Design review of the part built by this model. Coordinates are the model's own, in mm. A direction names the side the tool comes from. Give positions to 0.01 mm unless a question says otherwise; leave off trailing zeros. Write each loop counter-clockwise with the first axis right and the second up, starting at its lowest first coordinate (ties: lowest second). Pieces come first, ordered by that corner, then holes. Notation, with made-up numbers: (-38, 82.25) -> (16, 82.25) arc R24 cw to (16, 100.25) -> close; hole circle Ø9 at (-22.75, 15). An arc over 180 degrees is marked (long way). Answer as a JSON object with one key per item and string values.
```python
from build123d import *

# Parameters (mm, degrees)
ESQUISSE1_R        = 1.925
BOSS_EXTRU_1_DEPTH = 5


with BuildPart() as part:
    # Esquisse1 → Boss.-Extru.1 (new body)
    with BuildSketch(Plane.XY):
        with BuildLine():
            Line((13.05, 32.5), (-13.05, 32.5))
            ThreePointArc((-13.05, 32.5), (-14.464213562, 31.914213562), (-15.05, 30.5))
            Line((-15.05, 30.5), (-15.05, 25))
            Line((-15.05, 25), (-13.55, 25))
            Line((-13.55, 25), (-13.55, 21))
            Line((-13.55, 21), (-20.45, 21))
            Line((-20.45, 21), (-20.45, 25))
            Line((-20.45, 25), (-18.95, 25))
            Line((-18.95, 25), (-18.95, 30.5))
            ThreePointArc((-18.95, 30.5), (-19.535786438, 31.914213562), (-20.95, 32.5))
            Line((-20.95, 32.5), (-23, 32.5))
            Line((-23, 32.5), (-23, 37.5))
            Line((-23, 37.5), (-25.999999067, 37.497633905))
            ThreePointArc((-25.999999067, 37.497633905), (-26.620839292, 37.398317642), (-27.180168114, 37.111163374))
            ThreePointArc((-27.180168114, 37.111163374), (-45.999999844, 0), (-27.180168114, -37.111163374))
            ThreePointArc((-27.180168114, -37.111163374), (-26.620839292, -37.398317642), (-25.999999067, -37.497633905))
            Line((-25.999999067, -37.497633905), (-23, -37.5))
            Line((-23, -37.5), (-23, -32.5))
            Line((-23, -32.5), (-20.95, -32.5))
            ThreePointArc((-20.95, -32.5), (-19.535786438, -31.914213562), (-18.95, -30.5))
            Line((-18.95, -30.5), (-18.95, -25))
            Line((-18.95, -25), (-20.45, -25))
            Line((-20.45, -25), (-20.45, -21))
            Line((-20.45, -21), (-13.55, -21))
            Line((-13.55, -21), (-13.55, -25))
            Line((-13.55, -25), (-15.05, -25))
            Line((-15.05, -25), (-15.05, -30.5))
            ThreePointArc((-15.05, -30.5), (-14.464213562, -31.914213562), (-13.05, -32.5))
            Line((-13.05, -32.5), (13.05, -32.5))
            ThreePointArc((13.05, -32.5), (14.464213562, -31.914213562), (15.05, -30.5))
            Line((15.05, -30.5), (15.05, -25))
            Line((15.05, -25), (13.55, -25))
            Line((13.55, -25), (13.55, -21))
            Line((13.55, -21), (20.45, -21))
            Line((20.45, -21), (20.45, -25))
            Line((20.45, -25), (18.95, -25))
            Line((18.95, -25), (18.95, -30.5))
            ThreePointArc((18.95, -30.5), (19.535786438, -31.914213562), (20.95, -32.5))
            Line((20.95, -32.5), (23, -32.5))
            Line((23, -32.5), (23, -37.5))
            Line((23, -37.5), (25.999999067, -37.497633905))
            ThreePointArc((25.999999067, -37.497633905), (26.620839292, -37.398317642), (27.180168114, -37.111163374))
            ThreePointArc((27.180168114, -37.111163374), (45.999999844, 0), (27.180168114, 37.111163374))
            ThreePointArc((27.180168114, 37.111163374), (26.620839292, 37.398317642), (25.999999067, 37.497633905))
            Line((25.999999067, 37.497633905), (23, 37.5))
            Line((23, 37.5), (23, 32.5))
            Line((23, 32.5), (20.95, 32.5))
            ThreePointArc((20.95, 32.5), (19.535786438, 31.914213562), (18.95, 30.5))
            Line((18.95, 30.5), (18.95, 25))
            Line((18.95, 25), (20.45, 25))
            Line((20.45, 25), (20.45, 21))
            Line((20.45, 21), (13.55, 21))
            Line((13.55, 21), (13.55, 25))
            Line((13.55, 25), (15.05, 25))
            Line((15.05, 25), (15.05, 30.5))
            ThreePointArc((15.05, 30.5), (14.464213562, 31.914213562), (13.05, 32.5))
        make_face()
        with Locations((27.75, 0)):
            Circle(ESQUISSE1_R, mode=Mode.SUBTRACT)
        with Locations((-21.933137835, -17)):
            Circle(ESQUISSE1_R, mode=Mode.SUBTRACT)
        with Locations((-21.933137835, 17)):
            Circle(ESQUISSE1_R, mode=Mode.SUBTRACT)
        with Locations((14.500000149, -5)):
            Circle(ESQUISSE1_R, mode=Mode.SUBTRACT)
        with Locations((14.500000149, 5)):
            Circle(ESQUISSE1_R, mode=Mode.SUBTRACT)
        with Locations((-34.499999851, -5)):
            Circle(ESQUISSE1_R, mode=Mode.SUBTRACT)
        with Locations((-34.499999851, 5)):
            Circle(ESQUISSE1_R, mode=Mode.SUBTRACT)
        with BuildLine():
            Line((10.150000149, -10), (10.150000149, -2.6))
            ThreePointArc((10.150000149, -2.6), (10.735786586, -1.185786438), (12.150000149, -0.6))
            Line((12.150000149, -0.6), (16.500000149, -0.6))
            ThreePointArc((16.500000149, -0.6), (17.100000149, 0), (16.500000149, 0.6))
            Line((16.500000149, 0.6), (12.150000149, 0.6))
            ThreePointArc((12.150000149, 0.6), (10.735786586, 1.185786438), (10.150000149, 2.6))
            Line((10.150000149, 2.6), (10.150000149, 10))
            Line((10.150000149, 10), (-30.149999851, 10))
            Line((-30.149999851, 10), (-30.149999851, 2.6))
            ThreePointArc((-30.149999851, 2.6), (-30.735786289, 1.185786438), (-32.149999851, 0.6))
            Line((-32.149999851, 0.6), (-36.499999851, 0.6))
            ThreePointArc((-36.499999851, 0.6), (-37.099999851, 0), (-36.499999851, -0.6))
            Line((-36.499999851, -0.6), (-32.149999851, -0.6))
            ThreePointArc((-32.149999851, -0.6), (-30.735786289, -1.185786438), (-30.149999851, -2.6))
            Line((-30.149999851, -2.6), (-30.149999851, -10))
            Line((-30.149999851, -10), (10.150000149, -10))
        make_face(mode=Mode.SUBTRACT)
    extrude(amount=BOSS_EXTRU_1_DEPTH)


solid = part.part
```
(1) For faces 1 (the cylindrical face through (45.996, -0.604, 2.465)), 2 (the flat face through (0, -32.5, 2)), 3 (the flat face through (13.55, 23, 2)), 4 (the flat face through (-1, -16, 0)), 5 (the flat face through (-22, 32.5, 2)), list the 3-axis set-ups (+Z, -Z, +X, -X, +Y, -Y) from which the entire face can be reached by the end or side of a thin tool; tool diameter is ignored.
Here are the results:
{"face 1": "+Z, -Z, +X", "face 2": "+Z, -Z, -Y", "face 3": "+Z, -Z", "face 4": "-Z, +X, -X, +Y, -Y", "face 5": "+Z, -Z, +Y"}
(2) We need section D-D, the plane y = -8.5. State the section outline as (x, z) points.
Here are the results:
{"outline": "(-45.21, 0) -> (-30.15, 0) -> (-30.15, 5) -> (-45.21, 5) -> close; (10.15, 0) -> (45.21, 0) -> (45.21, 5) -> (10.15, 5) -> close"}
(3) We need section A-A, the plane x = -10. State the section outline as (y, z) points, then the cut area to 3 significant figures.
Here are the results:
{"outline": "(-32.5, 0) -> (-10, 0) -> (-10, 5) -> (-32.5, 5) -> close; (10, 0) -> (32.5, 0) -> (32.5, 5) -> (10, 5) -> close", "area": "225 mm²"}
(4) For line 1 along Y through (x, z) = (0.5, 3.35); line 2 along Y through (x, z) = (14, 4.15); line 3 along X through (y, z) = (31, 1.6), list the stretches that pass through material, from the lowest coordinate up.
Here are the results:
{"line 1": "y = -32.5 to -10, 10 to 32.5", "line 2": "y = -32.26 to -25, -21 to -6.86, -3.14 to -0.6, 0.6 to 3.14, 6.86 to 21, 25 to 32.26", "line 3": "x = -33.99 to -19.01, -14.99 to 14.99, 19.01 to 33.99"}
(5) We need section B-B, the plane y = 5. State the section outline as (x, z) points (3 decimals), then the cut area to 3 significant figures.
Here are the results:
{"outline": "(-45.727, 0) -> (-36.425, 0) -> (-36.425, 5) -> (-45.727, 5) -> close; (-32.575, 0) -> (-30.15, 0) -> (-30.15, 5) -> (-32.575, 5) -> close; (10.15, 0) -> (12.575, 0) -> (12.575, 5) -> (10.15, 5) -> close; (16.425, 0) -> (45.727, 0) -> (45.727, 5) -> (16.425, 5) -> close", "area": "217 mm²"}
(6) We need section C-C, the plane x = -34.5. State the section outline as (y, z) points (3 decimals), then the cut area to 3 significant figures.
Here are the results:
{"outline": "(-30.426, 0) -> (-6.925, 0) -> (-6.925, 5) -> (-30.426, 5) -> close; (-3.075, 0) -> (-0.6, 0) -> (-0.6, 5) -> (-3.075, 5) -> close; (0.6, 0) -> (3.075, 0) -> (3.075, 5) -> (0.6, 5) -> close; (6.925, 0) -> (30.426, 0) -> (30.426, 5) -> (6.925, 5) -> close", "area": "260 mm²"}
(7) The part is to be moulded in two halves that separate along Y. For faces 6 (the flat face through (0, 32.5, 2)), 7 (the flat face through (14, 0.6, 2)), 8 (the flat face through (-18.95, -28, 2)), say which applies: +Y half, -Y half, draft (parallel to the pull), parting line (faces both ways), or undercut.
Here are the results:
{"face 6": "+Y half", "face 7": "undercut", "face 8": "draft"}
(8) Clearance check with flat-ended pins moving along their axes: pin 1 (1.5 mm diameter, centred on x = 12, z = 2.5, fed in from -Y); pin 2 (2.5 mm diameter, centred on x = -5, z = 2.5, fed in from +Y); pin 3 (2.5 mm diameter, centred on x = -16.5, z = 3, fed in from +Y). State where each tip first meets the part, or that it passes through.
Here are the results:
{"pin 1": "stops at y = -32.5", "pin 2": "stops at y = 32.5", "pin 3": "stops at y = 21"}
